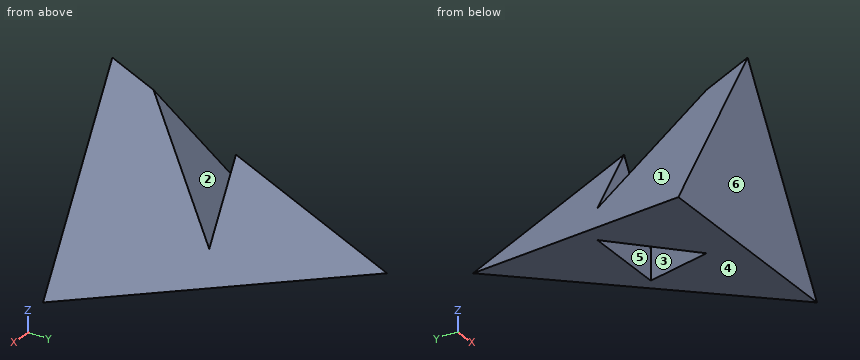
Autodesk Inventor part; units mm, degrees
ref_plane "РабПлоскость2" through (0, 100, 0) normal (0, 1, 0) x (-1, 0, 0)
ref_plane "YZ Plane" through (0, 0, 0) normal (1, 0, 0) x (0, 1, 0)
ref_plane "XY Plane" through (0, 0, 0) normal (0, 0, 1) x (1, 0, 0)
sketch "Эскиз1" plane through (0, 0, 0) normal (0, 1, 0) x (-1, 0, 0)
  line L0 (0, 45) -> (38.9711, -22.5)
  line L1 (38.9711, -22.5) -> (-38.9711, -22.5)
  line L2 (-38.9711, -22.5) -> (0, 45)
  point P0 (0, 0)
  point P1 (0, 0)
ref_plane "РабПлоскость2" through (0, 100, 0) normal (0, 1, 0) x (-1, 0, 0)
ref_plane "РабПлоскость1" through (0, 0, 0) normal (0, 1, 0) x (-1, 0, 0)
sketch "Эскиз2" plane through (0, 100, 0) normal (0, 1, 0) x (-1, 0, 0)
  point P0 (0, 0)
  point P1 (0, 0)
loft "Лофт1" add profiles "Эскиз1" section 2 point at (0, 100, 0)
sketch "Эскиз3" plane through (0, 0, 0) normal (0, 0, 1) x (1, 0, 0)
  point P0 (0, 0)
sketch "Эскиз4" plane through (0, 0, 0) normal (0, 0, 1) x (1, 0, 0)
  line L0 (0, 45) -> (15, 45)
  line L1 (15, 45) -> (-15, 45)
  line L2 (-15, 45) -> (0, 15)
  line L3 (15, 45) -> (0, 15)
  point P0 (0, 0)
extrude "Выдавливание1" cut sketch "Эскиз4" along normal through all both and the other way through all
properties part number "Задача №2"
CAD build for the part. Positions are in the model's coordinates, mm. Face numbers are marked on the shaded views. A direction names the side the tool comes from. Coordinates: 2 decimals unless noted, no trailing zeros. Loops run counter-clockwise (first coordinate to the right, second up) from the corner with the lowest first, then second, coordinate; pieces in that order, holes last. Notation, with made-up numbers: (53, -33.5) -> (89, -33.5) arc R12 cw to (89, -22.5) -> close; hole circle Ø6 at (68.5, 45). An arc over 180 degrees is marked (long way). One line per item, written item: value.
1. Slice it at D-D on y = 20. Write the cut outline in (x, z), and give its area (3 significant figures).
Answers:
outline: (-31.18, -18) -> (-2.5, -18) -> (-2.5, 31.67) -> close; (2.5, -18) -> (31.18, -18) -> (2.5, 31.67) -> close
area: 1,420 mm^2
2. Slice it at A-A on x = 11. Write the cut outline in (y, z) (3 decimals), and give its area (3 significant figures).
Answers:
outline: (0, -22.5) -> (37, -14.175) -> (37, 9.297) -> (0, 25.947) -> close; (45, -12.375) -> (71.774, -6.351) -> (45, 5.697) -> close
area: 1,570 mm^2
3. Drill centre lines: line 1 (X direction, y = 5, z = -12); line 2 (X direction, y = 47.5, z = 7.5); line 3 (Z direction, x = -11.5, y = 11.5). Where is each one in solid material? Low to high. Write a range as [from, to].
Answers:
line 1: x = [-31.61, 31.61]
line 2: x = [-9.31, 9.31]
line 3: z = [-19.91, 19.91]
4. Slice it at B-B on z = 15. Write the cut outline in (x, y).
Answers:
outline: (-17.32, 0) -> (17.32, 0) -> (8.83, 32.67) -> (0, 15) -> (-8.83, 32.67) -> close; (-5.63, 45) -> (5.63, 45) -> (0, 66.67) -> close
5. Slice it at C-C on z = -3. Write the cut outline in (x, y).
Answers:
outline: (-27.71, 0) -> (27.71, 0) -> (5.2, 86.67) -> (-5.2, 86.67) -> close; hole (-15, 45) -> (0, 15) -> (15, 45) -> close
6. Which spindle directions (+Z, -Z, +X, -X, +Y, -Y) get a long thin tool onto all of the face, cutting with end or side? Do the marked faces 1 and 2. Say none if no direction does.
Answers:
face 1: +Z, -X, +Y
face 2: +Z, -Z
7. Pull direction Y, two halves, no side cores. Call the marked faces 3, 4, 5 and 6: pulls with the +Y half, pulls with the -Y half, needs draft (parallel to the pull), parting line crosses it, or undercut.
Answers:
face 3: undercut
face 4: pulls with the +Y half
face 5: undercut
face 6: pulls with the -Y half
8. Flat gauge pins, fed straight in: P1, Ø5, axis at y = 38, z = 6, coming from the -X side; P2, Ø12, axis at x = 7, y = 11.5, coming from the +Z side; P3, Ø3, axis at y = 62.5, z = -9, coming from the +X side; P4, Ø24, axis at x = -1, z = -2, coming from the -Y side. Where does each tip first touch, or does it go through?
Answers:
P1: stops at x = -14.23
P2: stops at z = 38.44
P3: stops at x = 15.19
P4: stops at y = 0
